from build123d import *

# Parameters (mm, degrees)
SKETCH_1_W      = 230
SKETCH_1_H      = 600
SKETCH_1_R      = 2
SKETCH_1_W_2    = 150
SKETCH_1_H_2    = 570
EXTRUDE_1_DEPTH = 3


with BuildPart() as part:
    # 草图1 → 凸台-拉伸1 (new body)
    with BuildSketch(Plane(origin=(0, 0, 0), x_dir=(0, 0, -1), z_dir=(1, 0, 0))):
        Rectangle(SKETCH_1_W, SKETCH_1_H)
        with Locations((-107.5, 285)):
            Circle(SKETCH_1_R, mode=Mode.SUBTRACT)
        with Locations((-107.698004772, 210)):
            Circle(SKETCH_1_R, mode=Mode.SUBTRACT)
        with Locations((-107.5, -210)):
            Circle(SKETCH_1_R, mode=Mode.SUBTRACT)
        with Locations((-107.5, -285)):
            Circle(SKETCH_1_R, mode=Mode.SUBTRACT)
        with Locations((-107.698004772, 10)):
            Circle(SKETCH_1_R, mode=Mode.SUBTRACT)
        with Locations((107.5, -285)):
            Circle(SKETCH_1_R, mode=Mode.SUBTRACT)
        with Locations((107.5, -210)):
            Circle(SKETCH_1_R, mode=Mode.SUBTRACT)
        with Locations((107.698004772, 210)):
            Circle(SKETCH_1_R, mode=Mode.SUBTRACT)
        with Locations((107.5, 285)):
            Circle(SKETCH_1_R, mode=Mode.SUBTRACT)
        with Locations((107.698004772, 10)):
            Circle(SKETCH_1_R, mode=Mode.SUBTRACT)
        Rectangle(SKETCH_1_W_2, SKETCH_1_H_2, mode=Mode.SUBTRACT)
    extrude(amount=EXTRUDE_1_DEPTH)


solid = part.part
Can you work these out from the model? Positions are in its coordinate system, mm. Give positions to 0.01 mm unless a question says otherwise; leave off trailing zeros. Loops run counter-clockwise (first coordinate to the right, second up) from the corner with the lowest first, then second, coordinate; pieces in that order, holes last. Notation, with made-up numbers: (35.25, -30) -> (70.25, -30) arc R17 ccw to (70.25, 1) -> close; hole circle Ø1 at (-38.5, -27.75). An arc over 180 degrees is marked (long way). Return JSON: item names as keys, results as strings.
Q1. I need wall thicknesses on probe 1 along Z at (x, y) = (0.9, -210); probe 2 along Y at (x, z) = (1.8, 107.5); probe 3 along Z at (x, y) = (0.9, 210). Which ranges of each line are inside material? Lowest first, please.
Checks:
{"probe 1": "z = -115 to -109.5, -105.5 to -75, 75 to 105.5, 109.5 to 115", "probe 2": "y = -300 to -287, -283 to -212, -208 to 8.01, 11.99 to 208.01, 211.99 to 283, 287 to 300", "probe 3": "z = -115 to -109.7, -105.7 to -75, 75 to 105.7, 109.7 to 115"}
Q2. I want a section at A-A, the plane y = 241. List the corners of the cut face in (x, z) for me, then the cut area to 3 significant figures.
Checks:
{"outline": "(0, -115) -> (3, -115) -> (3, -75) -> (0, -75) -> close; (0, 75) -> (3, 75) -> (3, 115) -> (0, 115) -> close", "area": "240 mm2"}
Q3. I want a section at C-C, the plane x = 2.1. Count the separate pieces of the cut face and the enclosed holes in it, then the cut area to 3 significant figures.
Checks:
{"separate pieces": "1", "enclosed holes": "11", "area": "52,400 mm2"}
Q4. I want a section at B-B, the plane z = -26. List the corners of the cut face in (x, y) for me, then the cut area to 3 significant figures.
Checks:
{"outline": "(0, -300) -> (3, -300) -> (3, -285) -> (0, -285) -> close; (0, 285) -> (3, 285) -> (3, 300) -> (0, 300) -> close", "area": "90.0 mm2"}
Q5. For pin 1 Ø3 at (y, z) = (10, 107.7) entering from -X, with a flat end and sliding along its axis, tell me the tip position at first contact or that it passes through.
Checks:
{"pin 1": "passes through"}
